The listing builds one solid part. Answer for the finished solid, in the listing's coordinates (mm). A direction names the side the tool comes from. Coordinates: 2 decimals unless noted, no trailing zeros. Write each loop counter-clockwise with the first axis right and the second up, starting at its lowest first coordinate (ties: lowest second). Pieces come first, ordered by that corner, then holes.
```python
from build123d import *

# Parameters (mm, degrees)
SKETCH_W   = 100
SKETCH_H   = 50
SKETCH_W_2 = 25
SKETCH_H_2 = 40
PAD_DEPTH  = 20


with BuildPart() as part:
    # Sketch → Pad (new body)
    with BuildSketch(Plane.XY):
        with Locations((0.264387, 0.19665)):
            Rectangle(SKETCH_W, SKETCH_H)
        with Locations((-29.796774, -0.02574)):
            Rectangle(SKETCH_W_2, SKETCH_H_2, mode=Mode.SUBTRACT)
        with Locations((0.203226, -0.02574)):
            Rectangle(SKETCH_W_2, SKETCH_H_2, mode=Mode.SUBTRACT)
        with Locations((30.203226, -0.02574)):
            Rectangle(SKETCH_W_2, SKETCH_H_2, mode=Mode.SUBTRACT)
    extrude(amount=PAD_DEPTH)


solid = part.part
```
(1) Section A-A, the plane x = 39 is taken. Write down the section's boundary in (y, z).
(2) Section B-B, the plane y = -18.5 is taken. Write down the section's boundary in (x, z), plus the area to 3 significant figures.
(3) For a pull along Y with two mould halves and no side action, classify faces 3 (the flat face through (0, 25.197, 10)), 4 (the flat face through (-49.736, 0, 10)), 5 (the flat face through (-17.297, 0, 10)) as pulls with the +Y half, pulls with the -Y half, needs draft (parallel to the pull), parting line crosses it, or undercut.
(4) Which of the six approach directions +Z, -Z, +X, -X, +Y, -Y give full straight-line access (tool end or side, diameter ignored) to faces 1 (the flat face through (-30, -20.026, 10)), 2 (the flat face through (0, -24.803, 10))?
(5) Section C-C, the plane z = 9.5 is taken. Write down the section's boundary in (x, y).
(6) Find the intervals of material crossed by probe 1 along X at (y, z) = (-16, 11.25); probe 2 along Y at (x, z) = (11.5, 19.25), in increasing order.
Solution:
1. outline: (-24.8, 0) - (-20.03, 0) - (-20.03, 20) - (-24.8, 20) - close; (19.97, 0) - (25.2, 0) - (25.2, 20) - (19.97, 20) - close
2. outline: (-49.74, 0) - (-42.3, 0) - (-42.3, 20) - (-49.74, 20) - close; (-17.3, 0) - (-12.3, 0) - (-12.3, 20) - (-17.3, 20) - close; (12.7, 0) - (17.7, 0) - (17.7, 20) - (12.7, 20) - close; (42.7, 0) - (50.26, 0) - (50.26, 20) - (42.7, 20) - close
2. area: 500 mm2
3. face 3: pulls with the +Y half
3. face 4: needs draft
3. face 5: undercut
4. face 1: +Z, -Z
4. face 2: +Z, -Z, +X, -X, -Y
5. outline: (-49.74, -24.8) - (50.26, -24.8) - (50.26, 25.2) - (-49.74, 25.2) - close; hole (-42.3, -20.03) - (-17.3, -20.03) - (-17.3, 19.97) - (-42.3, 19.97) - close; hole (-12.3, -20.03) - (12.7, -20.03) - (12.7, 19.97) - (-12.3, 19.97) - close; hole (17.7, -20.03) - (42.7, -20.03) - (42.7, 19.97) - (17.7, 19.97) - close
6. probe 1: x = -49.74 to -42.3, -17.3 to -12.3, 12.7 to 17.7, 42.7 to 50.26
6. probe 2: y = -24.8 to -20.03, 19.97 to 25.2
